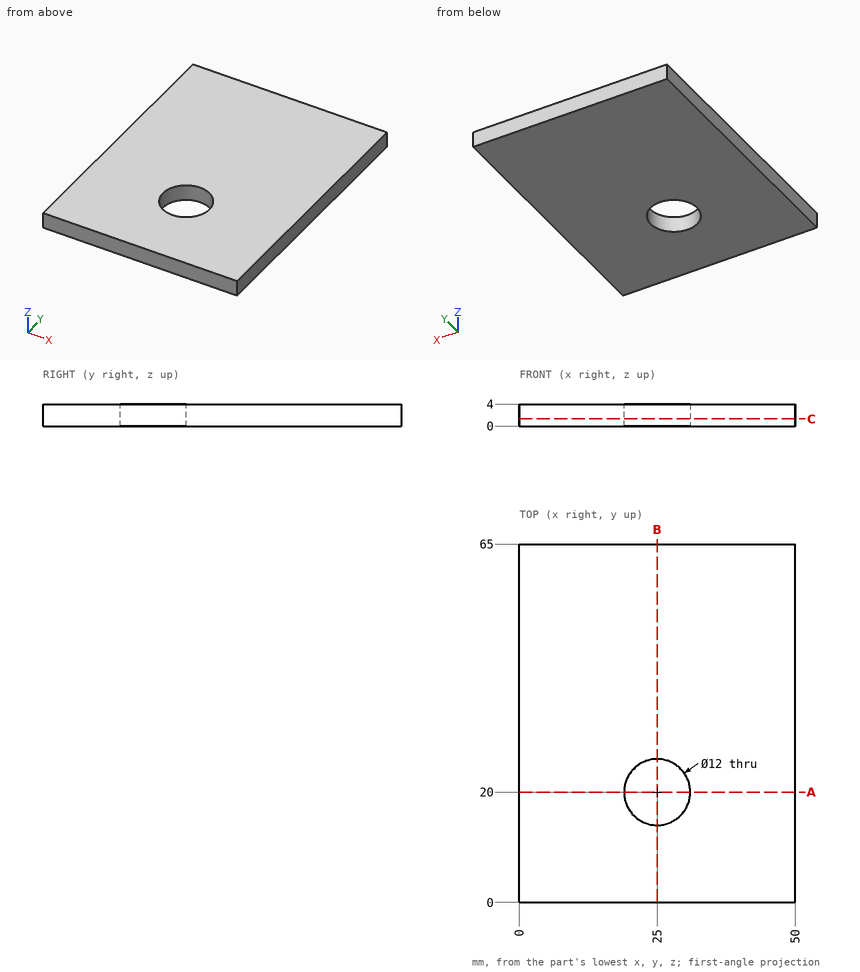
Design review of the part shown in the three views and the two pictorial views. Dimensions are in mm from the part's minimum x, y and z. Give positions to 0.01 mm unless a question says otherwise; leave off trailing zeros. Loops run counter-clockwise (first coordinate to the right, second up) from the corner with the lowest first, then second, coordinate; pieces in that order, holes last. Notation, with made-up numbers: (14.5, 39) -> (62.5, 39) arc R22 ccw to (62.5, 51) -> close; hole circle Ø1 at (79, 52). An arc over 180 degrees is marked (long way). One line per item, written item: value.
Q1. We need section C-C on z = 1.3. Give the boundary of the cut face in (x, y).
Numbers:
outline: (0, 0) -> (50, 0) -> (50, 65) -> (0, 65) -> close; hole circle Ø12 at (25, 20)
Q2. For pin 1 Ø1 at (y, z) = (58, 0.5) entering from -X, flat-tipped, find the tip position at first contact; note if it passes through.
Numbers:
pin 1: stops at x = 0
Q3. For L1, parallel to Y at x = 25, z = 0.9; L2, parallel to Y at x = 26, z = 1.7, list the stretches that pass through material, from the lowest coordinate up.
Numbers:
L1: y = 0 to 14, 26 to 65
L2: y = 0 to 14.08, 25.92 to 65
Q4. We need section A-A on y = 20. Give the boundary of the cut face in (x, z).
Numbers:
outline: (0, 0) -> (19, 0) -> (19, 4) -> (0, 4) -> close; (31, 0) -> (50, 0) -> (50, 4) -> (31, 4) -> close
Q5. We need section B-B on x = 25. Give the boundary of the cut face in (y, z).
Numbers:
outline: (0, 0) -> (14, 0) -> (14, 4) -> (0, 4) -> close; (26, 0) -> (65, 0) -> (65, 4) -> (26, 4) -> close
